```python
from build123d import *

# Parameters (mm, degrees)
F1_DEPTH = 25
F2_R     = 5


with BuildPart() as f1:
    # F0 (on Front) → F1 (new body)
    with BuildSketch(Plane.XZ):
        with BuildLine():
            Line((0, -51.609781), (0, 0))
            Line((0, 0), (-5, 0))
            Line((-5, 0), (-5, -51.609781))
            ThreePointArc((-5, -51.609781), (23.458993, -80.068774), (51.917986, -51.609781))
            Line((51.917986, -51.609781), (46.917986, -51.609781))
            ThreePointArc((46.917986, -51.609781), (23.458993, -75.068774), (0, -51.609781))
        make_face()
    extrude(amount=F1_DEPTH)

    # F2
    f2_edges = [f1.edges().sort_by_distance(p)[0] for p in [
        (49.417986, -25, -51.609781),
        (49.417986, 0, -51.609781),
        (-2.5, 0, 0),
        (-2.5, -25, 0),
    ]]
    fillet(f2_edges, radius=F2_R)


solid = f1.part
```
Geometry: final body of the model. Coordinates: model frame, mm. A direction names the side the tool comes from. Coordinates: 2 decimals unless noted, no trailing zeros. Loops run counter-clockwise (first coordinate to the right, second up) from the corner with the lowest first, then second, coordinate; pieces in that order, holes last. Notation, with made-up numbers: (87.25, -10) -> (141.25, -10) arc R12 cw to (141.25, 8) -> close; hole circle Ø8 at (36.5, 78). An arc over 180 degrees is marked (long way). Use a Markdown table: item, result. Add a question column.
(1) Access query for faces 4 (the flat face through (0, -12, -26)), 5 (the cylindrical face through (49.11, -1.5, -53.04)), 6 (the cylindrical face through (49.11, -23.5, -53.04)), 7 (the flat face through (2, -25, -62)), 8 (the cylindrical face through (-3, -2, -1)). Directions: +Z, -Z, +X, -X, +Y, -Y. A direction counts if a zero-diameter tool reaches every point of the face in a straight line with its end or side. Return the directions, or none.
(2) Line query: line 1 along X through (y, z) = (-5.5, -39); line 2 along X through (y, z) = (-16.75, -63); line 3 along X through (y, z) = (-4.25, -57.5). Output: solid intervals per line, ascending.
(3) Section query A-A, the plane z = -68. Return loops of the section in (x, y).
(4) Section query C-C, the plane x = 40.5. Return loops of the section in (y, z).
(5) Mould query, pull axis X, two halves, no side actions, for faces 1 (the cylindrical face through (22.83, -12.32, -80.06)), 2 (the flat face through (-2, -12, 0)), 3 (the cylindrical face through (23.975, -12.325, -75.063)). Classes: pulls with the +X half, pulls with the -X half, needs draft (parallel to the pull), parting line crosses it, or undercut.
(6) Section query D-D, the plane z = -44. Return loops of the section in (x, y), plus the area to 3 significant figures.
(7) Section query B-B, the plane y = -12. Return loops of the section in (x, z).
(8) Pin query (flat end, axial travel): pin 1 Ø5 at (x, y) = (32, -11) entering from -Z; pin 2 Ø10 at (x, y) = (6, -17.5) entering from -Z; pin 3 Ø7.5 at (y, z) = (-11.5, -13) entering from +X. Return the tip coordinate at first contact, or that it passes through.
Answer:
| question | item | result |
|---|---|---|
| 1 | face 4 | +Z, +X, +Y, -Y |
| 1 | face 5 | +Z, +X, +Y |
| 1 | face 6 | +Z, +X, -Y |
| 1 | face 7 | +Z, -Z, +X, -X, -Y |
| 1 | face 8 | +Z, +X, -X, +Y |
| 2 | line 1 | x = -5 to 0 |
| 2 | line 2 | x = -2.62 to 2.95, 43.97 to 49.54 |
| 2 | line 3 | x = -4.38 to 0.75, 46.17 to 51.3 |
| 3 | outline | (0.19, -25) -> (6.68, -25) -> (6.68, 0) -> (0.19, 0) -> close; (40.24, -25) -> (46.72, -25) -> (46.72, 0) -> (40.24, 0) -> close |
| 4 | outline | (-25, -74.4) -> (0, -74.4) -> (0, -67.73) -> (-25, -67.73) -> close |
| 5 | face 1 | parting line crosses it |
| 5 | face 2 | needs draft |
| 5 | face 3 | undercut |
| 6 | outline | (-5, -25) -> (0, -25) -> (0, 0) -> (-5, 0) -> close |
| 6 | area | 125 mm^2 |
| 7 | outline | (-5, -51.61) arc R28.46 ccw to (51.92, -51.61) -> (46.92, -51.61) arc R23.46 cw to (0, -51.61) -> (0, 0) -> (-5, 0) -> close |
| 8 | pin 1 | stops at z = -79.42 |
| 8 | pin 2 | stops at z = -77.2 |
| 8 | pin 3 | stops at x = 0 |
